The model under review builds one solid part; all positions refer to its coordinate system, in mm. Face numbers are marked on the shaded views. A direction names the side the tool comes from. Round coordinates to 2 decimals unless told otherwise and drop trailing zeros. Order: outer loops, then holes, each group sorted by start corner. A loop starts at its lowest first (then second) coordinate and runs counter-clockwise, first axis right, second up. Notation, with made-up numbers: M 87,39 L 146,39 A26 cw 146,58 Z; hole C 60,85.25 d7. An arc over 180 degrees is marked long. Use a Markdown table: item, result. Add a question column.
1. Consider section A-A on x = -1795.5. State the section outline as (y, z) points.
2. For the marked faces 4, 5, 6 and 7, list the 3-axis set-ups (+Z, -Z, +X, -X, +Y, -Y) from which the entire face can be reached by the end or side of a thin tool; tool diameter is ignored.
3. Consider section D-D on x = -1730.5. State the section outline as (y, z) points (3 decimals), then the cut area to 3 significant figures.
4. Insertion check: P1, Ø1.5, axis at x = -1835.5, z = -2828, coming from the +Y side; P2, Ø4, axis at y = 1615, z = -2827, coming from the -X side; P3, Ø1.5, axis at x = -1811.5, z = -2824.5, coming from the +Y side. Each pin has a flat end and moves straight along its axis. Give the tip position at first contact, or say it passes through.
5. Consider section C-C on z = -2824.75. Count the separate pieces of the cut face and the enclosed holes in it, then the cut area to 3 significant figures.
6. Consider section B-B on x = -1747.5. State the section outline as (y, z) points (3 decimals), then the cut area to 3 significant figures.
7. To check wall thickness, follow probe 1 along Y at (x, z) = (-1764.5, -2821); probe 2 along Y at (x, z) = (-1834, -2821.75); probe 3 along Y at (x, z) = (-1726.5, -2824.5). State the ranges of each line that lie inside material, in increasing order.
8. The part is to be moulded in two halves that separate along X. For the marked faces 1, 2 and 3, say which applies: +X half, -X half, draft (parallel to the pull), parting line (faces both ways), or undercut.
from build123d import *

# Parameters (mm, degrees)
BOSS_EXTRUDE1_DEPTH      = 8
BOSS_EXTRUDE1_DEPTH_BACK = 6
SKETCH1_R                = 36
SKETCH1_R_2              = 3.175
BOSS_EXTRUDE2_START      = -2
SKETCH3_R                = 36
SKETCH3_R_2              = 34.4
BOSS_EXTRUDE2_DEPTH      = 2
SKETCH4_R                = 3.175
CUT_EXTRUDE1_DEPTH       = 3267.782082753
FILLET11_R               = 12.7
CUT_EXTRUDE2_DEPTH       = 22.352
FILLET13_R               = 7.62
BOSS_EXTRUDE5_DEPTH      = 14
FILLET16_R               = 6.35
FILLET17_R               = 3.175
SKETCH10_W               = 14
SKETCH10_H               = 38.1
SKETCH10_R               = 3.175
SKETCH10_H_2             = 29.591
BOSS_EXTRUDE6_DEPTH      = 25.4
BOSS_EXTRUDE7_REACH      = 3394.349
SKETCH11_W               = 25.4
SKETCH11_H               = 14
FILLET18_R               = 5


with BuildPart() as part:
    # Sketch1 → Boss-Extrude1 (new, two sides: drawn at the far end of the back side and taken through both)
    with BuildSketch(Plane(origin=(-1819.591456758, 1585.913991712, -2825.111273399), x_dir=(1, 0, 0), z_dir=(0, 0, 1)).offset(-BOSS_EXTRUDE1_DEPTH_BACK)):
        with BuildLine():
            Line((2.684706364, 17.24642532), (66.819706364, 17.24642532))
            Line((66.819706364, 17.24642532), (66.819706364, 40.10642532))
            Line((66.819706364, 40.10642532), (76.344706364, 40.10642532))
            Line((76.344706364, 40.10642532), (76.344706364, 2.00642532))
            Line((76.344706364, 2.00642532), (39.954706364, -31.45357468))
            Line((39.954706364, -31.45357468), (76.344706364, -71.030146707))
            Line((76.344706364, -71.030146707), (76.344706364, -100.621146707))
            Line((76.344706364, -100.621146707), (66.819706364, -100.621146707))
            Line((66.819706364, -100.621146707), (66.819706364, -80.301146707))
            Line((66.819706364, -80.301146707), (-13.825293636, -80.301146707))
            ThreePointArc((-13.825293636, -80.301146707), (-16.969178238, -79.679037025), (-19.63920674, -77.906474293))
            Line((-19.63920674, -77.906474293), (-31.614211644, -66.026312835))
            ThreePointArc((-31.614211644, -66.026312835), (-42.345185642, -12.90636934), (2.684706364, 17.24642532))
        make_face()
        with Locations((2.684706364, -31.45357468)):
            Circle(SKETCH1_R, mode=Mode.SUBTRACT)
        with Locations((56.024706364, -72.046146707)):
            Circle(SKETCH1_R_2, mode=Mode.SUBTRACT)
        with Locations((-13.825293636, -72.046146707)):
            Circle(SKETCH1_R_2, mode=Mode.SUBTRACT)
    extrude(amount=BOSS_EXTRUDE1_DEPTH + BOSS_EXTRUDE1_DEPTH_BACK)

    # Sketch3 → Boss-Extrude2 (add)
    with BuildSketch(Plane.XY.offset(-2817.111273399).offset(BOSS_EXTRUDE2_START)):
        with Locations((-1816.906750395, 1554.460417032)):
            Circle(SKETCH3_R)
        with Locations((-1816.906750395, 1554.460417032)):
            Circle(SKETCH3_R_2, mode=Mode.SUBTRACT)
    extrude(amount=BOSS_EXTRUDE2_DEPTH)

    # Sketch4 → Cut-Extrude1 (cut, through all)
    with BuildSketch(Plane.ZY.offset(1752.771750395)):
        with Locations((-2824.111273399, 1618.400417032)):
            Circle(SKETCH4_R)
        with Locations((-2824.111273399, 1491.642845005)):
            Circle(SKETCH4_R)
    extrude(amount=-CUT_EXTRUDE1_DEPTH, mode=Mode.SUBTRACT)

    # Fillet11
    fillet11_edges = [part.edges().sort_by_distance(p)[0] for p in [
        (-1779.636750395, 1554.460417032, -2824.111273399),
    ]]
    fillet(fillet11_edges, radius=FILLET11_R)

    # Sketch6 → Cut-Extrude2 (cut)
    with BuildSketch(Plane(origin=(0, 0, -2831.111273399), x_dir=(-1, 0, 0), z_dir=(0, 0, -1))):
        with BuildLine():
            Line((1772.683835409, 1569.479812149), (1757.712123838, 1583.246052027))
            ThreePointArc((1757.712123838, 1583.246052027), (1756.093845604, 1590.22696014), (1762.010124746, 1594.270417032))
            Line((1762.010124746, 1594.270417032), (1789.841933512, 1594.270417032))
            ThreePointArc((1789.841933512, 1594.270417032), (1792.856665482, 1592.091417106), (1791.733381238, 1588.545309093))
            ThreePointArc((1791.733381238, 1588.545309093), (1783.527991751, 1580.529266005), (1777.768914276, 1570.608661686))
            ThreePointArc((1777.768914276, 1570.608661686), (1775.52091162, 1568.717450047), (1772.683835409, 1569.479812149))
        make_face()
        with BuildLine():
            Line((1782.693449915, 1521.233845005), (1764.944287612, 1521.233845005))
            ThreePointArc((1764.944287612, 1521.233845005), (1762.037080925, 1523.132610591), (1762.60710511, 1526.557845459))
            Line((1762.60710511, 1526.557845459), (1773.061547126, 1537.927754155))
            ThreePointArc((1773.061547126, 1537.927754155), (1775.907154759, 1538.912781284), (1778.29542193, 1537.07867628))
            ThreePointArc((1778.29542193, 1537.07867628), (1781.295178562, 1531.536772561), (1785.082430904, 1526.500111328))
            ThreePointArc((1785.082430904, 1526.500111328), (1785.584850577, 1523.097194437), (1782.693449915, 1521.233845005))
        make_face()
        Polygon((1824.186318893, 1512.343845005), (1784.281249696, 1512.343845005), (1764.963750395, 1505.612845005), (1752.771750395, 1505.612845005), (1752.771750395, 1485.292845005), (1829.340879649, 1505.612845005), align=None)
    extrude(amount=-CUT_EXTRUDE2_DEPTH, mode=Mode.SUBTRACT)

    # Fillet13
    fillet13_edges = [part.edges().sort_by_distance(p)[0] for p in [
        (-1752.771750395, 1603.160417032, -2824.111273399),
    ]]
    fillet(fillet13_edges, radius=FILLET13_R)

    # Sketch9 → Boss-Extrude5 (add)
    with BuildSketch(Plane.XY.offset(-2817.111273399)):
        Polygon((-1764.963750395, 1505.612845005), (-1752.771750395, 1505.612845005), (-1752.771750395, 1501.364657871), align=None)
    extrude(amount=-BOSS_EXTRUDE5_DEPTH)

    # Fillet16
    fillet16_edges = [part.edges().sort_by_distance(p)[0] for p in [
        (-1824.186318893, 1512.343845005, -2824.111273399),
        (-1829.340879649, 1505.612845005, -2824.111273399),
        (-1784.281249696, 1512.343845005, -2824.111273399),
    ]]
    fillet(fillet16_edges, radius=FILLET16_R)

    # Fillet17
    fillet17_edges = [part.edges().sort_by_distance(p)[0] for p in [
        (-1752.771750395, 1501.364657871, -2824.111273399),
    ]]
    fillet(fillet17_edges, radius=FILLET17_R)

    # Sketch10 → Boss-Extrude6 (add)
    # profile 1 of 2: a face of its own
    with BuildSketch(Plane(origin=(-1743.246750395, 0, 0), x_dir=(0, 0, -1), z_dir=(1, 0, 0))):
        with Locations((2824.111273399, 1606.970417032)):
            Rectangle(SKETCH10_W, SKETCH10_H)
        with Locations(Location((2824.111273399, 1618.400417032, 0), (0, 0, 180))):
            Circle(SKETCH10_R, mode=Mode.SUBTRACT)
    # profile 2 of 2: a face of its own
    with BuildSketch(Plane(origin=(-1743.246750395, 0, 0), x_dir=(0, 0, -1), z_dir=(1, 0, 0))):
        with Locations((2824.111273399, 1500.088345005)):
            Rectangle(SKETCH10_W, SKETCH10_H_2)
        with Locations(Location((2824.111273399, 1491.642845005, 0), (0, 0, 180))):
            Circle(SKETCH10_R, mode=Mode.SUBTRACT)
    extrude(amount=BOSS_EXTRUDE6_DEPTH)

    # Boss-Extrude7: up to this plane
    boss_extrude7_end = Plane(origin=(-1743.246750395, 1587.920417032, -2831.111273399), z_dir=(0.6768505367088385, -0.7361204731271623, 0))
    # Sketch11 → Boss-Extrude7 (add, up to the surface)
    with BuildSketch(Plane(origin=(0, 1514.883845005, 0), x_dir=(1, 0, 0), z_dir=(0, 1, 0)), mode=Mode.PRIVATE) as boss_extrude7_sk1:
        with Locations((-1730.546750395, 2824.111273399)):
            Rectangle(SKETCH11_W, SKETCH11_H)
    boss_extrude7_tool1 = split(extrude(boss_extrude7_sk1.sketch, amount=BOSS_EXTRUDE7_REACH, mode=Mode.PRIVATE), bisect_by=boss_extrude7_end, keep=Keep.BOTH, mode=Mode.PRIVATE)
    add(boss_extrude7_tool1.solids().sort_by_distance((-1730.54675, 1514.883845, -2824.111273))[0])

    # Fillet18
    fillet18_edges = [part.edges().sort_by_distance(p)[0] for p in [
        (-1743.246750395, 1587.920417032, -2824.111273399),
        (-1743.246750395, 1514.883845005, -2824.111273399),
    ]]
    fillet(fillet18_edges, radius=FILLET18_R)


solid = part.part
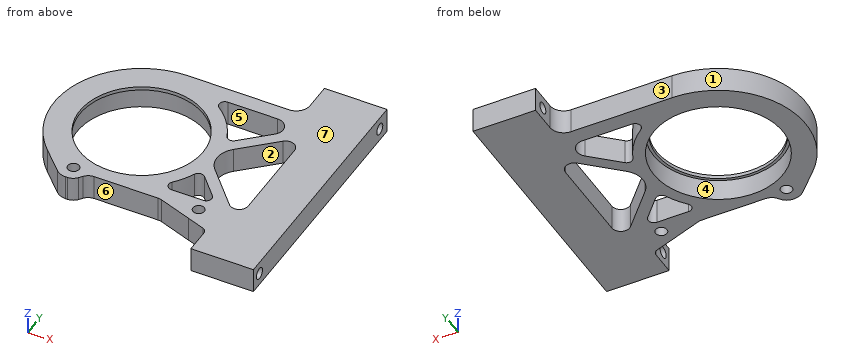
Answer block:
| question | item | result |
|---|---|---|
| 1 | outline | M 1512.34,-2831.11 L 1525.52,-2831.11 L 1525.52,-2819.11 L 1527.53,-2819.11 L 1527.53,-2817.11 L 1512.34,-2817.11 Z; M 1581.39,-2819.11 L 1583.4,-2819.11 L 1583.4,-2831.11 L 1603.16,-2831.11 L 1603.16,-2817.11 L 1581.39,-2817.11 Z |
| 2 | face 4 | -Z |
| 2 | face 5 | +Z, -Z |
| 2 | face 6 | +Z, -Z, -Y |
| 2 | face 7 | +Z, +X, -X, +Y, -Y |
| 3 | outline | M 1485.293,-2831.111 L 1626.02,-2831.111 L 1626.02,-2817.111 L 1485.293,-2817.111 Z; hole C 1491.643,-2824.111 d6.35; hole C 1618.4,-2824.111 d6.35 |
| 3 | area | 1,910 mm^2 |
| 4 | P1 | y = 1599.77 |
| 4 | P2 | x = -1752.77 |
| 4 | P3 | y = 1603.16 |
| 5 | separate pieces | 3 |
| 5 | enclosed holes | 6 |
| 5 | area | 7,970 mm^2 |
| 6 | outline | M 1485.293,-2831.111 L 1522.765,-2831.111 L 1522.765,-2817.111 L 1485.293,-2817.111 Z; M 1581.475,-2831.111 L 1626.02,-2831.111 L 1626.02,-2817.111 L 1581.475,-2817.111 Z; hole C 1491.643,-2824.111 d6.35; hole C 1618.4,-2824.111 d6.35 |
| 6 | area | 1,080 mm^2 |
| 7 | probe 1 | 1505.45 to 1510.83, 1516.9 to 1521.27, 1528.62 to 1538, 1568.38 to 1577, 1594.27 to 1603.16 |
| 7 | probe 2 | 1505.63 to 1510.75, 1516.99 to 1522.78, 1586.14 to 1600.06 |
| 7 | probe 3 | 1485.29 to 1488.49, 1494.79 to 1615.25, 1621.55 to 1626.02 |
| 8 | face 1 | -X half |
| 8 | face 2 | undercut |
| 8 | face 3 | draft |
